from build123d import *

# Parameters (mm, degrees)
SKETCH1_W           = 26
SKETCH1_H           = 12
BOSS_EXTRUDE1_DEPTH = 1
BOSS_EXTRUDE2_DEPTH = 9
BOSS_EXTRUDE3_DEPTH = 12
FILLET1_R           = 10


with BuildPart() as part:
    # Sketch1 → Boss-Extrude1 (new body)
    with BuildSketch(Plane(origin=(0, 0, 0), x_dir=(1, 0, 0), z_dir=(0, 1, 0))):
        with BuildLine():
            Line((-18, -12.5), (-18, 12.5))
            ThreePointArc((-18, 12.5), (0, 30.5), (18, 12.5))
            Line((18, 12.5), (18, -12.5))
            ThreePointArc((18, -12.5), (0, -30.5), (-18, -12.5))
        make_face()
        with Locations((0, 10.5)):
            Rectangle(SKETCH1_W, SKETCH1_H, mode=Mode.SUBTRACT)
    extrude(amount=BOSS_EXTRUDE1_DEPTH)

    # Sketch2 → Boss-Extrude2 (add)
    with BuildSketch(Plane(origin=(0, 0, 0), x_dir=(1, 0, 0), z_dir=(0, 1, 0))):
        with BuildLine():
            Line((20, -12.5), (20, 12.5))
            ThreePointArc((20, 12.5), (0, 32.5), (-20, 12.5))
            Line((-20, 12.5), (-20, -12.5))
            ThreePointArc((-20, -12.5), (0, -32.5), (20, -12.5))
        make_face()
        with BuildLine():
            Line((18, -12.5), (18, 12.5))
            ThreePointArc((18, 12.5), (0, 30.5), (-18, 12.5))
            Line((-18, 12.5), (-18, -12.5))
            ThreePointArc((-18, -12.5), (0, -30.5), (18, -12.5))
        make_face(mode=Mode.SUBTRACT)
    extrude(amount=BOSS_EXTRUDE2_DEPTH)

    # Sketch3 → Boss-Extrude3 (add, along a direction that is not the sketch's normal)
    with BuildSketch(Plane.XZ):
        Polygon((-20, 0), (0, 8.284271247), (20, 0), (20, 2.164784401), (0, 10.449055648), (-20, 2.164784401), align=None)
        Polygon((-20, -3.247176601), (0, 5.037094647), (20, -3.247176601), (20, -5.411961001), (0, 2.872310246), (-20, -5.411961001), align=None)
    extrude(amount=BOSS_EXTRUDE3_DEPTH, dir=(0, -0.9659258262890672, -0.25881904510252496))

    # Fillet1
    fillet1_edges = [part.edges().sort_by_distance(p)[0] for p in [
        (0, -5.795554958, 6.731356977),
        (0, -5.795554958, 8.896141377),
        (0, -5.795554958, 1.319395975),
        (0, -5.795554958, 3.484180376),
    ]]
    fillet(fillet1_edges, radius=FILLET1_R)


solid = part.part
Read the model definition and answer for the solid it produces. Units are mm, in the model's axes. A direction names the side the tool comes from. Coordinates: 2 decimals unless noted, no trailing zeros. Order: outer loops, then holes, each group sorted by start corner. A loop starts at its lowest first (then second) coordinate and runs counter-clockwise, first axis right, second up. Notation, with made-up numbers: M -32.75,-29.5 L -1.75,-29.5 A28 cw -1.75,8.5 Z; hole C 32.25,84 d6. An arc over 180 degrees is marked long. Put each result on its own line as item: value. Start each with the question number.
Item 1: Consider probe 1 along X at (y, z) = (4.25, -4); probe 2 along X at (y, z) = (0.25, -6.5); probe 3 along Y at (x, z) = (17, 16.5). Determine where each line is inside the solid, lowest interval first. Write a range as [from, to].
Item 2: Section D-D, the plane x = -16 is taken. Determine the outline of the cut face in (y, z).
Item 3: Section C-C, the plane z = 17 is taken. Determine the outline of the cut face in (x, y), plus the area to 3 significant figures.
Item 4: For faces 1 (the face through (-0.396, 4.944, 30.496)), 2 (the face through (-11.7, -5.7, -3.5)), 3 (the face through (0.053, -5.939, 5.895)), determine the directions among +Z, -Z, +X, -X, +Y, -Y from which every point of the face is accessible in a straight line to the end or side of a thin tool.
Item 5: The mould has two halves that part along X. Classify faces 4 (the face through (-0.1, 0, 4.5)), 5 (the face through (-20, 3, 0)), 6 (the face through (-0.44, 4.437, 32.495)): +X half, -X half, draft (parallel to the pull), parting line (faces both ways), or undercut.
Item 6: Section A-A, the plane x = -3 is taken. Determine the outline of the cut face in (y, z), plus the area to 3 significant figures.
Item 7: Section B-B, the plane y = 5.25 is taken. Determine the outline of the cut face in (x, z), plus the area to 3 significant figures.
Item 8: Given pin 1 Ø1.1 at (y, z) = (0.5, -13.5) entering from -X; pin 2 Ø4 at (x, y) = (4, 3.5) entering from +Z; pin 3 Ø5 at (x, z) = (14.5, 11) entering from -Y, each flat-ended and moving along its own axis, determine where each tip first touches the part or whether it passes through.
Computed:
1. probe 1: x = [-20, -18], [18, 20]
1. probe 2: x = [-20, -13], [13, 20]
1. probe 3: y = [0, 1]
2. outline: M -11.59,-6.86 L 0,-3.76 L 0,-24.5 L 9,-24.5 L 9,-20.75 L 1,-20.75 L 1,20.75 L 9,20.75 L 9,24.5 L 0,24.5 L 0,3.82 L -11.59,0.72 L -11.59,-1.45 L 0,1.66 L 0,-1.59 L -11.59,-4.7 Z
3. outline: M -19.49,0 L 19.49,0 L 19.49,9 L 17.43,9 L 17.43,1 L -17.43,1 L -17.43,9 L -19.49,9 Z
3. area: 71.9 mm2
4. face 1: +Y
4. face 2: -Z
4. face 3: none
5. face 4: undercut
5. face 5: -X half
5. face 6: parting line
6. outline: M -11.59,-1.51 L 0,1.6 L 0,-4.5 L 1,-4.5 L 1,30.25 L 9,30.25 L 9,32.27 L 0,32.27 L 0,9.17 L -11.59,6.07 L -11.59,3.9 L 0,7.01 L 0,3.76 L -11.59,0.66 Z; M 0,-32.27 L 9,-32.27 L 9,-30.25 L 1,-30.25 L 1,-16.5 L 0,-16.5 Z
6. area: 135 mm2
7. outline: M -20,-12.5 A20 ccw 20,-12.5 L 20,12.5 A20 ccw -20,12.5 Z; hole M -18,-12.5 A18 ccw 18,-12.5 L 18,12.5 A18 ccw -18,12.5 Z
7. area: 339 mm2
8. pin 1: stops at x = -19.99
8. pin 2: stops at z = 32.4
8. pin 3: stops at y = 0
